from build123d import *

# Parameters (mm, degrees)
BOSS_EXTRUDE1_DEPTH      = 12
BOSS_EXTRUDE2_START      = -2
BOSS_EXTRUDE2_DEPTH      = 2
SKETCH4_W                = 6
SKETCH4_H                = 4.8
BOSS_EXTRUDE3_DEPTH      = 20
BOSS_EXTRUDE4_DEPTH      = 3
BOSS_EXTRUDE4_DEPTH_BACK = 1.5
SKETCH5_W                = 18
SKETCH5_H                = 15
CUT_EXTRUDE1_DEPTH       = 5


with BuildPart() as part:
    # Sketch1 → Boss-Extrude1 (new body)
    with BuildSketch(Plane(origin=(0, 0, 0), x_dir=(1, 0, 0), z_dir=(0, 1, 0))):
        with BuildLine():
            Line((2.5, 27.386127875), (2.5, 25.377155081))
            ThreePointArc((2.5, 25.377155081), (25.5, 0), (2.5, -25.377155081))
            Line((2.5, -25.377155081), (2.5, -27.386127875))
            ThreePointArc((2.5, -27.386127875), (27.5, 0), (2.5, 27.386127875))
        make_face()
    extrude(amount=BOSS_EXTRUDE1_DEPTH)

    # Sketch2 → Boss-Extrude2 (add)
    with BuildSketch(Plane(origin=(0, 0, 0), x_dir=(1, 0, 0), z_dir=(0, 1, 0)).offset(BOSS_EXTRUDE2_START)):
        with BuildLine():
            Line((2.5, 27.386127875), (1.863636364, 20.415113507))
            ThreePointArc((1.863636364, 20.415113507), (20.5, 0), (1.863636364, -20.415113507))
            Line((1.863636364, -20.415113507), (2.5, -27.386127875))
            ThreePointArc((2.5, -27.386127875), (27.5, 0), (2.5, 27.386127875))
        make_face()
    extrude(amount=BOSS_EXTRUDE2_DEPTH)

    # Sketch4 → Boss-Extrude3 (add)
    with BuildSketch(Plane(origin=(0, -2, 0), x_dir=(1, 0, 0), z_dir=(0, 1, 0))):
        with Locations((30, 0)):
            Rectangle(SKETCH4_W, SKETCH4_H)
    extrude(amount=BOSS_EXTRUDE3_DEPTH)

    # Sketch5 → Boss-Extrude4 (add, two sides: drawn at the far end of the back side and taken through both)
    with BuildSketch(Plane(origin=(0, 18, 0), x_dir=(1, 0, 0), z_dir=(0, 1, 0)).offset(-BOSS_EXTRUDE4_DEPTH_BACK)):
        with Locations((24, 0)):
            Rectangle(SKETCH5_W, SKETCH5_H)
    extrude(amount=BOSS_EXTRUDE4_DEPTH + BOSS_EXTRUDE4_DEPTH_BACK)

    # Sketch6 → Cut-Extrude1 (cut)
    with BuildSketch(Plane(origin=(0, 21, 0), x_dir=(1, 0, 0), z_dir=(0, 1, 0))):
        with BuildLine():
            Line((24, -7.5), (15, -7.5))
            Line((15, -7.5), (15, 2.5))
            ThreePointArc((15, 2.5), (21.433067029, -0.760239674), (24, -7.5))
        make_face()
    extrude(amount=-CUT_EXTRUDE1_DEPTH, mode=Mode.SUBTRACT)


solid = part.part
Work out the finished part from the listing and answer in its coordinate system (mm). A direction names the side the tool comes from. Round coordinates to 2 decimals unless told otherwise and drop trailing zeros. Order: outer loops, then holes, each group sorted by start corner. A loop starts at its lowest first (then second) coordinate and runs counter-clockwise, first axis right, second up. Notation, with made-up numbers: M 82,-24.5 L 141,-24.5 A22 ccw 141,8.5 Z; hole C -7,34 d5. An arc over 180 degrees is marked long. Put each result on its own line as item: value. Start each with the question number.
Q1. Section A-A, the plane x = 4 is taken. Write down the section's boundary in (y, z), and give its area (3 significant figures).
Q2. Flat-ended cylindrical pins translate along their axes: pin 1 (3.5 mm diameter, centred on y = 19, z = -5.5, fed in from -X); pin 2 (5 mm diameter, centred on x = 26.5, y = 5.5, fed in from +Z); pin 3 (12 mm diameter, centred on x = 5.5, z = -7, fed in from +Y); pin 4 (2 mm diameter, centred on y = 7, z = 26, fed in from -X). Find the tip coordinate at first contact, or state that the pin passes through.
Q3. Straight lines are drawn through the part: L1, parallel to Y at x = 17, z = 15.5; L2, parallel to X at y = 15, z = 1; L3, parallel to X at y = 6, z = 0. For each, find the intervals that lie inside material, in ascending order. Write a range as [from, to].
Q4. Section B-B, the plane y = 8 is taken. Write down the section's boundary in (x, z).
Q5. A tool of negligible diameter and unlimited length cuts with its end or side. For faces 1 (the flat face through (24, 19, -7.5)), 2 (the flat face through (28, 19, 7.5)), 3 (the flat face through (21, 0, 0)), 4 (the cylindrical face through (20.496, -1.014, -0.425)), from which of +Z, -Z, +X, -X, +Y, -Y can it reach the whole face along a straight path? Write none if from no direction.
Q6. For a pull along Z with two mould halves and no side action, classify faces 5 (the flat face through (26, 16.5, -2)), 6 (the flat face through (2.177, -1.014, 23.852)), 7 (the cylindrical face through (25.495, 5.916, -0.526)) as pulls with the +Z half, pulls with the -Z half, needs draft (parallel to the pull), parting line crosses it, or undercut.
Q7. Section D-D, the plane x = 28 is taken. Write down the section's boundary in (y, z), and give its area (3 significant figures).
Q8. Section C-C, the plane z = -4 is taken. Write down the section's boundary in (x, y).
Findings below:
1. outline: M -2,-27.21 L 12,-27.21 L 12,-25.18 L 0,-25.18 L 0,-20.11 L -2,-20.11 Z; M -2,20.11 L 0,20.11 L 0,25.18 L 12,25.18 L 12,27.21 L -2,27.21 Z
1. area: 77.0 mm^2
2. pin 1: stops at x = 15
2. pin 2: stops at z = 13.43
2. pin 3: passes through
2. pin 4: stops at x = 2.5
3. L1: y = [-2, 0]
3. L2: x = [27, 33]
3. L3: x = [25.5, 33]
4. outline: M 2.5,-27.39 A27.5 ccw 27.4,-2.4 L 33,-2.4 L 33,2.4 L 27.4,2.4 A27.5 ccw 2.5,27.39 L 2.5,25.38 A25.5 cw 2.5,-25.38 Z
5. face 1: -Z, +X, -X, +Y
5. face 2: +Z, +X, -X, +Y
5. face 3: -X
5. face 4: -X, -Y
6. face 5: needs draft
6. face 6: pulls with the +Z half
6. face 7: undercut
7. outline: M -2,-2.4 L 16.5,-2.4 L 16.5,-7.5 L 21,-7.5 L 21,7.5 L 16.5,7.5 L 16.5,2.4 L -2,2.4 Z
7. area: 156 mm^2
8. outline: M 15,16.5 L 33,16.5 L 33,21 L 15,21 Z; M 20.11,-2 L 27.21,-2 L 27.21,12 L 25.18,12 L 25.18,0 L 20.11,0 Z
